```python
from build123d import *

# Parameters (mm, degrees)
F0_R      = 1.6
F1_DEPTH  = 1
F3_DEPTH  = 14
F2_W      = 1.4
F2_H      = 4.8
F4_DEPTH  = 12.5
F5_R      = 5
F6_DEPTH  = 1.8
F7_R      = 1
F8_DEPTH  = 1.7
F9_R      = 3
F10_DEPTH = 10
F11_W     = 4.6
F11_H     = 10.5
F12_DEPTH = 5


with BuildPart() as f1:
    # F0 (on Top) → F1 (new body)
    with BuildSketch(Plane.XY):
        with BuildLine():
            Line((15.5043796111, -8.1156769819), (15.5043796111, 8.1156769819))
            ThreePointArc((15.5043796111, 8.1156769819), (0, 17.5), (-15.5043796111, 8.1156769819))
            Line((-15.5043796111, 8.1156769819), (-15.5043796111, -8.1156769819))
            ThreePointArc((-15.5043796111, -8.1156769819), (0, -17.5), (15.5043796111, -8.1156769819))
        make_face()
        with BuildLine():
            Line((22.650669435, 2.7119651303), (15.5043796111, 8.1156769819))
            ThreePointArc((15.5043796111, 8.1156769819), (16.8286129371, 4.8008110372), (17.4526699029, 1.2862010962))
            ThreePointArc((17.4526699029, 1.2862010962), (19.700629708, 3.2788920504), (22.650669435, 2.7119651303))
        make_face()
        with BuildLine():
            ThreePointArc((17.4526699029, 1.2862010962), (16.8286129371, 4.8008110372), (15.5043796111, 8.1156769819))
            Line((15.5043796111, 8.1156769819), (15.5043796111, -8.1156769819))
            ThreePointArc((15.5043796111, -8.1156769819), (16.8286129371, -4.8008110372), (17.4526699029, -1.2862010962))
            ThreePointArc((17.4526699029, -1.2862010962), (17.2, 0), (17.4526699029, 1.2862010962))
        make_face()
        with BuildLine():
            Line((-15.5043796111, -8.1156769819), (-15.5043796111, 8.1156769819))
            ThreePointArc((-15.5043796111, 8.1156769819), (-16.8286129371, 4.8008110372), (-17.4526699029, 1.2862010962))
            ThreePointArc((-17.4526699029, 1.2862010962), (-17.2637654212, 0.655392123), (-17.2, 0))
            ThreePointArc((-17.2, 0), (-17.2637654212, -0.655392123), (-17.4526699029, -1.2862010962))
            ThreePointArc((-17.4526699029, -1.2862010962), (-16.8286129371, -4.8008110372), (-15.5043796111, -8.1156769819))
        make_face()
        with BuildLine():
            ThreePointArc((-17.4526699029, 1.2862010962), (-16.8286129371, 4.8008110372), (-15.5043796111, 8.1156769819))
            Line((-15.5043796111, 8.1156769819), (-22.650669435, 2.7119651303))
            ThreePointArc((-22.650669435, 2.7119651303), (-19.700629708, 3.2788920504), (-17.4526699029, 1.2862010962))
        make_face()
        with BuildLine():
            ThreePointArc((22.650669435, 2.7119651303), (19.700629708, 3.2788920504), (17.4526699029, 1.2862010962))
            ThreePointArc((17.4526699029, 1.2862010962), (17.4881634728, 0.6435358184), (17.5, 0))
            ThreePointArc((17.5, 0), (17.4881634728, -0.6435358184), (17.4526699029, -1.2862010962))
            ThreePointArc((17.4526699029, -1.2862010962), (19.700629708, -3.2788920504), (22.650669435, -2.7119651303))
            Line((22.650669435, -2.7119651303), (22.650669435, 2.7119651303))
        make_face()
        with Locations((20.6, 0)):
            Circle(F0_R, mode=Mode.SUBTRACT)
        with BuildLine():
            ThreePointArc((17.4526699029, -1.2862010962), (16.8286129371, -4.8008110372), (15.5043796111, -8.1156769819))
            Line((15.5043796111, -8.1156769819), (22.650669435, -2.7119651303))
            ThreePointArc((22.650669435, -2.7119651303), (19.700629708, -3.2788920504), (17.4526699029, -1.2862010962))
        make_face()
        with BuildLine():
            ThreePointArc((24, 0), (23.6440331863, 1.5145500851), (22.650669435, 2.7119651303))
            Line((22.650669435, 2.7119651303), (22.650669435, -2.7119651303))
            ThreePointArc((22.650669435, -2.7119651303), (23.6440331863, -1.5145500851), (24, 0))
        make_face()
        with BuildLine():
            ThreePointArc((-17.4526699029, -1.2862010962), (-17.5, 0), (-17.4526699029, 1.2862010962))
            ThreePointArc((-17.4526699029, 1.2862010962), (-19.700629708, 3.2788920504), (-22.650669435, 2.7119651303))
            Line((-22.650669435, 2.7119651303), (-22.650669435, -2.7119651303))
            ThreePointArc((-22.650669435, -2.7119651303), (-19.700629708, -3.2788920504), (-17.4526699029, -1.2862010962))
        make_face()
        with Locations((-20.6, 0)):
            Circle(F0_R, mode=Mode.SUBTRACT)
        with BuildLine():
            Line((-22.650669435, -2.7119651303), (-22.650669435, 2.7119651303))
            ThreePointArc((-22.650669435, 2.7119651303), (-24, 0), (-22.650669435, -2.7119651303))
        make_face()
        with BuildLine():
            Line((-22.650669435, -2.7119651303), (-15.5043796111, -8.1156769819))
            ThreePointArc((-15.5043796111, -8.1156769819), (-16.8286129371, -4.8008110372), (-17.4526699029, -1.2862010962))
            ThreePointArc((-17.4526699029, -1.2862010962), (-19.700629708, -3.2788920504), (-22.650669435, -2.7119651303))
        make_face()
        with BuildLine():
            ThreePointArc((-17.2, 0), (-17.2637654212, 0.655392123), (-17.4526699029, 1.2862010962))
            ThreePointArc((-17.4526699029, 1.2862010962), (-17.5, 0), (-17.4526699029, -1.2862010962))
            ThreePointArc((-17.4526699029, -1.2862010962), (-17.2637654212, -0.655392123), (-17.2, 0))
        make_face()
        with BuildLine():
            ThreePointArc((17.5, 0), (17.4881634728, 0.6435358184), (17.4526699029, 1.2862010962))
            ThreePointArc((17.4526699029, 1.2862010962), (17.2, 0), (17.4526699029, -1.2862010962))
            ThreePointArc((17.4526699029, -1.2862010962), (17.4881634728, -0.6435358184), (17.5, 0))
        make_face()
    extrude(amount=F1_DEPTH)

    # F2 (on face) → F3 (join)
    with BuildSketch(Plane.XY.offset(1)):
        with BuildLine():
            ThreePointArc((15.5043796111, -8.1156769819), (16.9937730242, -4.1787173155), (17.5, 0))
            ThreePointArc((17.5, 0), (16.9937730242, 4.1787173155), (15.5043796111, 8.1156769819))
            ThreePointArc((15.5043796111, 8.1156769819), (0, 17.5), (-15.5043796111, 8.1156769819))
            ThreePointArc((-15.5043796111, 8.1156769819), (-17.5, 0), (-15.5043796111, -8.1156769819))
            ThreePointArc((-15.5043796111, -8.1156769819), (-11.1280694067, -13.5061493875), (-5, -16.7705098312))
            Line((-5, -16.7705098312), (-5, 0))
            Line((-5, 0), (5, 0))
            Line((5, 0), (5, -16.7705098312))
            ThreePointArc((5, -16.7705098312), (11.1280694067, -13.5061493875), (15.5043796111, -8.1156769819))
        make_face()
        with BuildLine():
            ThreePointArc((-5.71e-08, -17.5), (2.5264676594, -17.3166671495), (5, -16.7705098312))
            Line((5, -16.7705098312), (5, 0))
            Line((5, 0), (-5, 0))
            Line((-5, 0), (-5, -16.7705098312))
            ThreePointArc((-5, -16.7705098312), (-2.5264677159, -17.3166671412), (-5.71e-08, -17.5))
        make_face()
    extrude(amount=F3_DEPTH)

    # F2 (on face) → F4 (join)
    with BuildSketch(Plane.XY.offset(1)):
        with BuildLine():
            ThreePointArc((5, -16.7705098312), (14.0312152004, -10.4582503317), (17.5, 0))
            ThreePointArc((17.5, 0), (-10.4582503317, 14.0312152004), (-5, -16.7705098312))
            Line((-5, -16.7705098312), (-5, 0))
            Line((-5, 0), (5, 0))
            Line((5, 0), (5, -16.7705098312))
        make_face()
        with BuildLine():
            Line((-5, 0), (-5, -16.7705098312))
            ThreePointArc((-5, -16.7705098312), (-2.5264677035, -17.316667143), (-3.21e-08, -17.5))
            ThreePointArc((-3.21e-08, -17.5), (2.5264676717, -17.3166671477), (5, -16.7705098312))
            Line((5, -16.7705098312), (5, 0))
            Line((5, 0), (-5, 0))
        make_face()
        with BuildLine():
            ThreePointArc((-3.21e-08, -17.5), (-2.5264677035, -17.316667143), (-5, -16.7705098312))
            Line((-5, -16.7705098312), (-5, -17.5))
            Line((-5, -17.5), (-3.21e-08, -17.5))
        make_face()
        with BuildLine():
            Line((5, -17.5), (5, -16.7705098312))
            ThreePointArc((5, -16.7705098312), (2.5264676717, -17.3166671477), (-3.21e-08, -17.5))
            Line((-3.21e-08, -17.5), (5, -17.5))
        make_face()
        Polygon((5, -17.5), (-3.21e-08, -17.5), (-5, -17.5), (-5, -22.3), (5, -22.3), align=None)
        Polygon((-5, -22.3), (-5, -17.5), (-8.4841037169, -17.5), (-21.1, -17.5), (-21.1, -22.3), align=None)
        with Locations((5.7, -19.9)):
            Rectangle(F2_W, F2_H)
        Polygon((-21.1, -17.5), (-8.4841037169, -17.5), (-16.5028385818, -11.7), (-21.1, -11.7), align=None)
    extrude(amount=F4_DEPTH)

    # F5 (on face) → F6 (join)
    with BuildSketch(Plane.XY.offset(15)):
        Circle(F5_R)
    extrude(amount=F6_DEPTH)

    # F7 (on face) → F8 (join)
    with BuildSketch(Plane.XY.offset(16.8)):
        Circle(F7_R)
    extrude(amount=F8_DEPTH)

    # F9 (on face) → F10 (join)
    with BuildSketch(Plane.XY.offset(18.5)):
        Circle(F9_R)
    extrude(amount=F10_DEPTH)

    # F11 (on face) → F12 (cut)
    with BuildSketch(Plane(origin=(-21.1, 0, 0), x_dir=(0, -1, 0), z_dir=(-1, 0, 0))):
        with Locations((15, 7.25)):
            Rectangle(F11_W, F11_H)
    extrude(amount=-F12_DEPTH, mode=Mode.SUBTRACT)


solid = f1.part
```
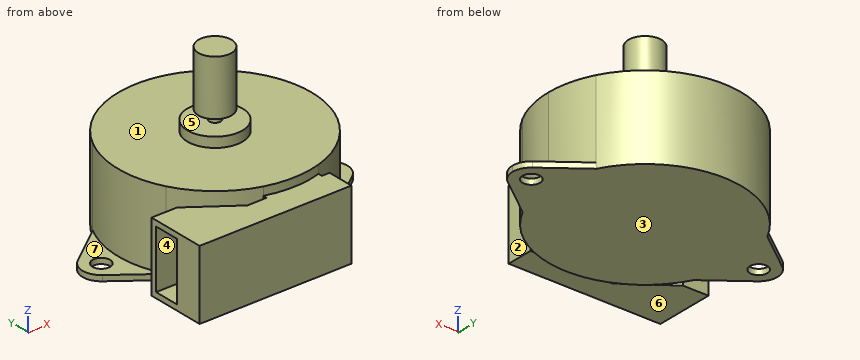
Work out the finished part from the listing and answer in its coordinate system (mm). Face numbers are marked on the shaded views. A direction names the side the tool comes from. Give positions to 0.01 mm unless a question says otherwise; leave off trailing zeros. Loops run counter-clockwise (first coordinate to the right, second up) from the corner with the lowest first, then second, coordinate; pieces in that order, holes last. Notation, with made-up numbers: (18.5, 31.25) - (58.5, 31.25) arc R31 ccw to (58.5, 56.25) - close; hole circle Ø6 at (-23.75, 28). An arc over 180 degrees is marked (long way). One line per question, with ' | ' between items.
(1) Straight lines are drawn through the part: probe 1 along Z at (x, y) = (-1, 2); probe 2 along Z at (x, y) = (2, -16); probe 3 along Z at (x, y) = (3.5, -19). For each, find the intervals that lie inside material, in ascending order.
Recorded:
probe 1: z = 0 to 16.8, 18.5 to 28.5 | probe 2: z = 0 to 15 | probe 3: z = 1 to 13.5
(2) The part is cut by section C-C (z = 6). Write down the section's boundary in (x, y).
Recorded:
outline: (-21.1, -22.3) - (6.4, -22.3) - (6.4, -17.5) - (5, -17.5) - (5, -16.77) arc R17.5 ccw (long way) to (-5, -16.77) - (-5, -17.5) - (-8.48, -17.5) - (-16.5, -11.7) - (-21.1, -11.7) - (-21.1, -12.7) - (-16.1, -12.7) - (-16.1, -17.3) - (-21.1, -17.3) - close
(3) A tool of negligible diameter and unlimited length cuts with its end or side. For the marked faces 1, 2 and 3, from which of +Z, -Z, +X, -X, +Y, -Y can it reach the whole face along a straight path? Write none if from no direction.
Recorded:
face 1: +Z | face 2: +Z, -Z, +X, -Y | face 3: -Z, +X, -X, +Y, -Y
(4) Each of these flat-tipped pins is pushed along its axis until it touches: pin 1 Ø4 at (x, z) = (-6, 6.5) entering from +Y; pin 2 Ø11.5 at (x, y) = (-6.5, -17) entering from -Z; pin 3 Ø10 at (y, z) = (-11.5, 24) entering from -X; pin 4 Ø9.5 at (x, y) = (21.5, 2) entering from +Z. Where does it stop, or does it pass through?
Recorded:
pin 1: stops at y = 17.04 | pin 2: stops at z = 0 | pin 3: passes through | pin 4: stops at z = 15
(5) The part is cut by section A-A (x = 0). Write down the section's boundary in (y, z).
Recorded:
outline: (-22.3, 1) - (-17.5, 1) - (-17.5, 0) - (17.5, 0) - (17.5, 15) - (5, 15) - (5, 16.8) - (1, 16.8) - (1, 18.5) - (3, 18.5) - (3, 28.5) - (-3, 28.5) - (-3, 18.5) - (-1, 18.5) - (-1, 16.8) - (-5, 16.8) - (-5, 15) - (-17.5, 15) - (-17.5, 13.5) - (-22.3, 13.5) - close
(6) The part is cut by section D-D (x = -7). Write down the section's boundary in (y, z).
Recorded:
outline: (-22.3, 1) - (-17.5, 1) - (-17.5, 13.5) - (-22.3, 13.5) - close; (-16.04, 0) - (16.04, 0) - (16.04, 15) - (-16.04, 15) - close
(7) The mould has two halves that part along Z. Classify the marked faces 4, 5, 6 and 7: +Z half, -Z half, draft (parallel to the pull), parting line (faces both ways), or undercut.
Recorded:
face 4: undercut | face 5: undercut | face 6: -Z half | face 7: +Z half
(8) The part is cut by section B-B (x = 20.6). Write down the section's boundary in (y, z), then the cut area to 3 significant figures.
Recorded:
outline: (-4.26, 0) - (-1.6, 0) - (-1.6, 1) - (-4.26, 1) - close; (1.6, 0) - (4.26, 0) - (4.26, 1) - (1.6, 1) - close | area: 5.33 mm²
